Autodesk Inventor part; units mm, degrees
ref_plane "YZ Plane" through (0, 0, 0) normal (1, 0, 0) x (0, 1, 0)
ref_plane "XZ Plane" through (0, 0, 0) normal (0, 1, 0) x (-1, 0, 0)
ref_plane "XY Plane" through (0, 0, 0) normal (0, 0, 1) x (1, 0, 0)
sketch "Sketch1" plane through (0, 0, 0) normal (0, 1, 0) x (-1, 0, 0)
  line L0 (0, 0) -> (25, 0)
  line L1 (25, 0) -> (25, -60)
  line L2 (25, -60) -> (0, -60)
  line L3 (0, -60) -> (0, 0)
  circle A0 centre (12.5, -4) radius 2
  circle A1 centre (12.5, -56) radius 2
  dimension "d0" = 25
  dimension "d1" = 60
  dimension "d2" = 4
  dimension "d3" = 4
  dimension "d4" = 52
  dimension "d5" = 4
extrude "Extrusion1" add sketch "Sketch1" along normal blind 7
sketch "Sketch2" plane through (0, 7, 0) normal (0, 1, 0) x (1, 0, 0)
  line L0 (-25, 60) -> (-25, 0)
  line L1 (-25, 25) -> (0, 25)
  line L2 (0, 25) -> (0, 35)
  line L3 (0, 35) -> (-25, 35)
  line L4 (-25, 35) -> (-25, 25)
  line L5 (0, 60) -> (-25, 60)
  point P0 (0, 0)
  dimension "d8" = 25
  dimension "d9" = 10
  dimension "d10" = 25
extrude "Extrusion2" add sketch "Sketch2" along normal blind 20
sketch "Sketch3" plane through (-25, 7, -25) normal (0, 0, 1) x (1, 0, 0)
  circle A0 centre (12.5, 10) radius 5
  line L0 (2, 15.0299) -> (5.5, 15.0299)
  line L1 (5.5, 15.0299) -> (5.5, 5.0299)
  line L2 (5.5, 5.0299) -> (2, 5.0299)
  line L3 (2, 5.0299) -> (2, 15.0299)
  line L4 (19.5, 15.0299) -> (23, 15.0299)
  line L5 (23, 15.0299) -> (23, 5.0299)
  line L6 (23, 5.0299) -> (19.5, 5.0299)
  line L7 (19.5, 5.0299) -> (19.5, 15.0299)
  line L8 (0, 0) -> (0, 20)
  point P0 (25, -7)
  dimension "d13" = 10
  dimension "d14" = 3.5
  dimension "d15" = 10
  dimension "d16" = 3.5
  dimension "d17" = 10
  dimension "d20" = 7
  dimension "d21" = 7
  dimension "d22" = 12.5
extrude "Extrusion3" cut sketch "Sketch3" against normal blind 20
sketch "Sketch4" plane through (0, 0, 0) normal (1, 0, 0) x (0, 0, -1)
  line L0 (-8.0858, 30.1503) -> (63.6355, 30.1503)
  line L1 (63.6355, 30.1503) -> (63.6355, -9.4106)
  line L2 (63.6355, -9.4106) -> (-8.0858, -9.4106)
  line L3 (-8.0858, -9.4106) -> (-8.0858, 30.1503)
  point P0 (0, 0)
extrude "Extrusion4" cut sketch "Sketch4" against normal blind 5.5
properties part number "zthreadedrod"
Geometry: final body of the model. Coordinates: model frame, mm. A direction names the side the tool comes from. Coordinates: 2 decimals unless noted, no trailing zeros. Order: outer loops, then holes, each group sorted by start corner. A loop starts at its lowest first (then second) coordinate and runs counter-clockwise, first axis right, second up.
1) Section A-A (z = -56). Return loops of the section in (x, y).
Result sheet:
outline: (-25, 0) - (-14.5, 0) - (-14.5, 7) - (-25, 7) - close; (-10.5, 0) - (-5.5, 0) - (-5.5, 7) - (-10.5, 7) - close
2) Section C-C (y = 17). Return loops of the section in (x, z).
Result sheet:
outline: (-25, -35) - (-23, -35) - (-23, -25) - (-25, -25) - close; (-19.5, -35) - (-17.5, -35) - (-17.5, -25) - (-19.5, -25) - close; (-7.5, -35) - (-5.5, -35) - (-5.5, -25) - (-7.5, -25) - close
3) Draft query along Z for faces 1 (the flat face through (-18, 17, -25)), 2 (the cylindrical face through (-10.9, 3.5, -2.8)), 3 (the cylindrical face through (-12.24, 3.451, -57.983)), 4 (the flat face through (-23, 17, -30)). Return one class per face: released by +Z, released by -Z, zero draft, split by the parting line, or undercut.
Result sheet:
face 1: released by +Z
face 2: undercut
face 3: undercut
face 4: zero draft
4) Section B-B (x = -12.5). Return loops of the section in (y, z), then the cut area to 3 significant figures.
Result sheet:
outline: (0, -60) - (7, -60) - (7, -58) - (0, -58) - close; (0, -54) - (7, -54) - (7, -35) - (12, -35) - (12, -25) - (7, -25) - (7, -6) - (0, -6) - close; (0, -2) - (7, -2) - (7, 0) - (0, 0) - close; (22, -35) - (27, -35) - (27, -25) - (22, -25) - close
area: 464 mm2
5) First-contact query: P1, Ø3, axis at x = -17, y = 21, coming from the +Z side; P2, Ø6, axis at x = -13, y = 12, coming from the -Z side; P3, Ø6, axis at x = -17.5, z = -7.5, coming from the +Y side. Flat tips, straight axial feed; report the tip coordinate or a pass-through.
Result sheet:
P1: stops at z = -25
P2: stops at z = -35
P3: stops at y = 7
6) Set-up query: faces 5 (the flat face through (-15, 7, -12)), 6 (the flat face through (-19.5, 17, -30)), 7 (the flat face through (-15, 3, 0)), 8 (the flat face through (-17.3, 14.6, -35)). Return all of +Z, -Z, +X, -X, +Y, -Y with unobstructed straight access to the full face (end or side cutting, diameter ignored); none if empty.
Result sheet:
face 5: +Z, +X, -X, +Y
face 6: +Z, -Z
face 7: +Z, +X, -X, +Y, -Y
face 8: -Z, +X, -X, +Y
7) Ray query, probe 1 along Z at (x, y) = (-12.5, 2); probe 2 along Y at (x, z) = (-20, -33); probe 3 along Y at (x, z) = (-22.5, -7). Return the intervals inside material, ascending.
Result sheet:
probe 1: z = -60 to -58, -54 to -6, -2 to 0
probe 2: y = 0 to 12.03, 22.03 to 27
probe 3: y = 0 to 7
8) Section D-D (x = -6.75). Return loops of the section in (y, z), then the cut area to 3 significant figures.
Result sheet:
outline: (0, -60) - (7, -60) - (7, -35) - (27, -35) - (27, -25) - (7, -25) - (7, 0) - (0, 0) - close
area: 620 mm2
